The model under review builds one solid part; all positions refer to its coordinate system, in mm. A direction names the side the tool comes from. Round coordinates to 2 decimals unless told otherwise and drop trailing zeros. Write each loop counter-clockwise with the first axis right and the second up, starting at its lowest first coordinate (ties: lowest second). Pieces come first, ordered by that corner, then holes. Notation, with made-up numbers: M 87.5,-23.5 L 145.5,-23.5 A5 cw 145.5,-17.5 Z; hole C 50,-10.75 d7. An arc over 180 degrees is marked long. Write item = value, one per line. Start each with the question number.
Item 1: The part is to be moulded in two halves that separate along Y. For faces 3 (the cylindrical face through (-8.968, -457.915, -0.14)), 4 (the flat face through (-8, -448, -10)), say which applies: +Y half, -Y half, draft (parallel to the pull), parting line (faces both ways), or undercut.
Item 2: Tool access review of faces 1 (the flat face through (-8, 0, 10)), 2 (the cylindrical face through (-3.71, -220.99, -0.52)): name each direction out of +Z, -Z, +X, -X, +Y, -Y from which nothing blocks a thin tool from reaching the whole face with its end or side.
Item 3: Take a section at B-B, the plane y = -385.5. Give the boundary of the cut face in (x, z), plus the area to 3 significant figures.
Item 4: For pin 1 Ø5 at (x, y) = (-8.5, -362) entering from -Z; pin 2 Ø10 at (x, z) = (-0.5, -6.5) entering from +Y; pin 3 Ø12 at (y, z) = (-66.5, -1) entering from -X, all flat-tipped, find the tip position at first contact; note any pin that passes through.
Item 5: Take a section at A-A, the plane z = 0. Give the boundary of the cut face in (x, y), plus the area to 3 significant figures.
Item 6: To check wall thickness, follow line 1 along Y through (x, z) = (-6.75, 3.75); line 2 along Y through (x, z) = (-13, -0.75); line 3 along X through (y, z) = (-30, 0). State the ranges of each line that lie inside material, in increasing order.
from build123d import *

# Parameters (mm, degrees)
SKETCH1_R                = 5
BOSS_EXTRUDE1_DEPTH      = 80
BOSS_EXTRUDE2_DEPTH      = 10
BOSS_EXTRUDE2_DEPTH_BACK = 10
SKETCH2_R                = 10
SKETCH3_R                = 3.98820793
BOSS_EXTRUDE3_DEPTH      = 450


with BuildPart() as part:
    # Sketch1 → Boss-Extrude1 (new body)
    with BuildSketch(Plane(origin=(0, 0, 0), x_dir=(0, 0, -1), z_dir=(1, 0, 0))):
        Circle(SKETCH1_R)
    extrude(amount=BOSS_EXTRUDE1_DEPTH)


with BuildPart() as body_2:
    # Sketch2 → Boss-Extrude2 (new, two sides: drawn at the far end of the back side and taken through both)
    with BuildSketch(Plane.XY.offset(-BOSS_EXTRUDE2_DEPTH_BACK)):
        with Locations((-7.666034923, 0)):
            Circle(SKETCH2_R)
    extrude(amount=BOSS_EXTRUDE2_DEPTH + BOSS_EXTRUDE2_DEPTH_BACK)


with BuildPart() as body_3:
    # Mirror1: mirrored copy
    add(part.part.mirror(Plane.ZX.offset(-224)))


with BuildPart() as body_4:
    # Mirror1 2: mirrored copy
    add(body_2.part.mirror(Plane.ZX.offset(-224)))


with BuildPart() as body_2_1:
    add(body_2.part)

    add(body_4.part)  # Boss-Extrude3 merges body 4
    # Sketch3 → Boss-Extrude3 (add)
    with BuildSketch(Plane(origin=(0, 0, 0), x_dir=(1, 0, 0), z_dir=(0, 1, 0))):
        with Locations(Location((-7.666034923, 0, 0), (0, 0, 270))):
            Circle(SKETCH3_R)
    extrude(amount=-BOSS_EXTRUDE3_DEPTH)


solid = body_2_1.part
Response values:
q1.face_3 = undercut
q1.face_4 = draft
q2.face_1 = +Z, +X, -X, +Y, -Y
q2.face_2 = none
q3.outline = C -7.67,0 d7.98
q3.area = 50.0 mm2
q4.pin_1 = -3.99
q4.pin_2 = 9.76
q4.pin_3 = -11.65
q5.outline = M -11.65,-438.83 A10 ccw long -3.68,-438.83 L -3.68,-9.17 A10 ccw long -11.65,-9.17 Z
q5.area = 4,050 mm2
q6.line_1 = -457.96 to 9.96
q6.line_2 = -456.46 to -439.54, -8.46 to 8.46
q6.line_3 = -11.65 to -3.68
